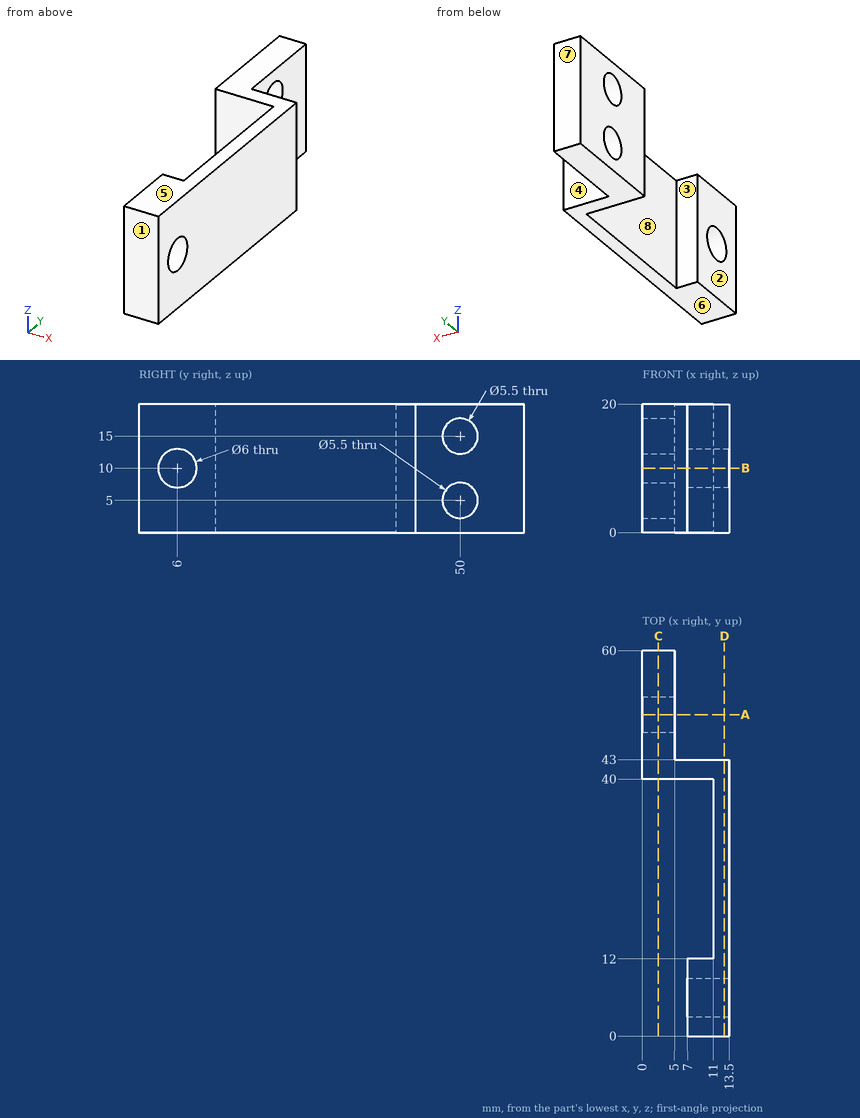
Drawing for the job (mm, zero at the part's lowest x, y, z). A direction names the side the tool comes from. Round coordinates to 2 decimals unless told otherwise and drop trailing zeros. Order: outer loops, then holes, each group sorted by start corner. A loop starts at its lowest first (then second) coordinate and runs counter-clockwise, first axis right, second up. Notation, with made-up numbers: (-17, 52.5) -> (21, 52.5) arc R22 ccw to (21, 81.5) -> close; hole circle Ø11 at (5, 76). An arc over 180 degrees is marked (long way). Write item = value, one per line. Start each with the question number.
(1) Cut at B-B, the plane z = 10. List the corners of the cut face in (x, y), then the cut area to 4 significant figures.
(2) Cut at D-D, the plane x = 12.75. List the corners of the cut face in (y, z).
(3) Which spindle directions (+Z, -Z, +X, -X, +Y, -Y) get a long thin tool onto all of the face, cutting with end or side? Do the marked faces 1, 2, 3, 4 and 5. Say none if no direction does.
(4) Pin check, flat tips, straight feed: P1, Ø4, axis at x = 8.5, z = 6.5, coming from the +Y side; P2, Ø8, axis at x = 4.5, z = 5, coming from the -Y side; P3, Ø8.5, axis at y = 49, z = 7.5, coming from the +X side; P4, Ø3.5, axis at y = 50, z = 5, coming from the -X side. Stop position of each tip, or through.
(5) Cut at C-C, the plane x = 2.5. List the corners of the cut face in (y, z).
(6) Probe line 1 (Y direction, x = 10.25, z = 10); line 2 (Y direction, x = 1.25, z = 4.75); line 3 (Y direction, x = 9.75, z = 16.5). List the from-to ranges inside material, lowest first. Write a range as [from, to].
(7) Pull direction Y, two halves, no side cores. Call the marked faces 6, 7 and 8: released by +Y, released by -Y, zero draft, split by the parting line, or undercut.
(8) Cut at A-A, the plane y = 50. List the corners of the cut face in (x, z).
Model answer:
q1.outline = (0, 40) -> (11, 40) -> (11, 12) -> (7, 12) -> (7, 9) -> (13.5, 9) -> (13.5, 43) -> (5, 43) -> (5, 60) -> (0, 60) -> close; (7, 0) -> (13.5, 0) -> (13.5, 3) -> (7, 3) -> close
q1.area = 234.5 mm2
q2.outline = (0, 0) -> (43, 0) -> (43, 20) -> (0, 20) -> close; hole circle Ø6 at (6, 10)
q3.face_1 = +Z, -Z, +X, -X, -Y
q3.face_2 = +Z, -Z, -X, -Y
q3.face_3 = +Z, -Z, -X
q3.face_4 = +Z, -Z, +X, +Y
q3.face_5 = +Z, +X, -X, +Y, -Y
q4.P1 = 43
q4.P2 = 0
q4.P3 = 5
q4.P4 = through
q5.outline = (40, 0) -> (60, 0) -> (60, 20) -> (40, 20) -> close; hole circle Ø5.5 at (50, 5); hole circle Ø5.5 at (50, 15)
q6.line_1 = [0, 3], [9, 12], [40, 43]
q6.line_2 = [40, 47.26], [52.74, 60]
q6.line_3 = [0, 12], [40, 43]
q7.face_6 = zero draft
q7.face_7 = released by +Y
q7.face_8 = undercut
q8.outline = (0, 0) -> (5, 0) -> (5, 2.25) -> (0, 2.25) -> close; (0, 7.75) -> (5, 7.75) -> (5, 12.25) -> (0, 12.25) -> close; (0, 17.75) -> (5, 17.75) -> (5, 20) -> (0, 20) -> close
